CAD build for the part. Positions are in the model's coordinates, mm. Face numbers are marked on the shaded views. A direction names the side the tool comes from. Round coordinates to 2 decimals unless told otherwise and drop trailing zeros. Loops run counter-clockwise (first coordinate to the right, second up) from the corner with the lowest first, then second, coordinate; pieces in that order, holes last.
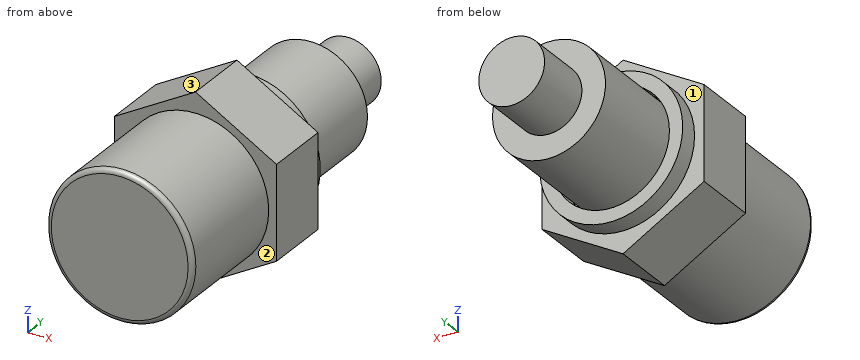
from build123d import *

# Parameters (mm, degrees)
F0_R      = 3.45
F1_DEPTH  = 6.3
F2_R      = 5.925
F3_DEPTH  = 12.5
F5_DEPTH  = 7
F6_R      = 7.675
F7_DEPTH  = 12.8
F8_R      = 0.5
F9_R      = 7.5
F9_R_2    = 6.107803
F10_DEPTH = 2


with BuildPart() as f1:
    # F0 (on Front) → F1 (new body)
    with BuildSketch(Plane.XZ):
        Circle(F0_R)
    extrude(amount=F1_DEPTH)

    # F2 (on face) → F3 (join)
    with BuildSketch(Plane.XZ.offset(6.3)):
        Circle(F2_R)
    extrude(amount=F3_DEPTH)

    # F4 (on face) → F5 (join)
    with BuildSketch(Plane.XZ.offset(18.8)):
        Polygon((0, 9.814955), (-8.5, 4.907477), (-8.5, -4.907477), (0, -9.814955), (8.5, -4.907477), (8.5, 4.907477), align=None)
    extrude(amount=F5_DEPTH)

    # F6 (on face) → F7 (join)
    with BuildSketch(Plane.XZ.offset(25.8)):
        Circle(F6_R)
    extrude(amount=F7_DEPTH)

    # F8
    f8_edges = [f1.edges().sort_by_distance(p)[0] for p in [
        (-7.675, -38.6, 0),
    ]]
    fillet(f8_edges, radius=F8_R)

    # F9 (on face) → F10 (join)
    with BuildSketch(Plane(origin=(0, -18.8, 0), x_dir=(-1, 0, 0), z_dir=(0, 1, 0))):
        Circle(F9_R)
        Circle(F9_R_2, mode=Mode.SUBTRACT)
    extrude(amount=F10_DEPTH)


solid = f1.part
Item 1: Wall check: L1, parallel to Z at x = 0, y = -18.1 (3 decimals); L2, parallel to X at y = -18.5, z = 2; L3, parallel to Y at x = 5.25, z = 0.75. Give the ranges that are in metal, low to high.
Verdict:
L1: z = -7.5 to -6.108, -5.925 to 5.925, 6.108 to 7.5
L2: x = -7.23 to -5.77, -5.58 to 5.58, 5.77 to 7.23
L3: y = -38.6 to -6.3
Item 2: Cut at C-C (y = -13). List the corners of the cut face in (x, z) (3 decimals).
Verdict:
outline: circle Ø11.85 at (0, 0)
Item 3: Cut at B-B (y = -25). List the corners of the cut face in (x, z), plus the area to 3 significant figures.
Verdict:
outline: (-8.5, -4.91) - (0, -9.81) - (8.5, -4.91) - (8.5, 4.91) - (0, 9.81) - (-8.5, 4.91) - close
area: 250 mm2
Item 4: Cut at A-A (z = 0). List the corners of the cut face in (x, y) (3 decimals).
Verdict:
outline: (-8.5, -25.8) - (-7.675, -25.8) - (-7.675, -38.1) arc R0.5 ccw to (-7.175, -38.6) - (7.175, -38.6) arc R0.5 ccw to (7.675, -38.1) - (7.675, -25.8) - (8.5, -25.8) - (8.5, -18.8) - (7.5, -18.8) - (7.5, -16.8) - (6.108, -16.8) - (6.108, -18.8) - (5.925, -18.8) - (5.925, -6.3) - (3.45, -6.3) - (3.45, 0) - (-3.45, 0) - (-3.45, -6.3) - (-5.925, -6.3) - (-5.925, -18.8) - (-6.108, -18.8) - (-6.108, -16.8) - (-7.5, -16.8) - (-7.5, -18.8) - (-8.5, -18.8) - close
Item 5: 3-axis set-ups, long thin cutter, end or side, ignore diameter. For the marked faces 1, 2 and 3: which of +Z, -Z, +X, -X, +Y, -Y reach the whole face in a straight line?
Verdict:
face 1: +Y
face 2: -Y
face 3: +Z, -X, +Y, -Y
Item 6: Flat gauge pins, fed straight in: P1, Ø1, axis at x = 6, y = -10.5, coming from the -Z side; P2, Ø5, axis at x = 2.5, y = -34, coming from the +Z side (3 decimals); P3, Ø4, axis at x = -6, z = 8, coming from the -Y side. Where does each tip first touch, or does it go through?
Verdict:
P1: stops at z = -2.2
P2: stops at z = 7.675
P3: stops at y = -25.8
